The figure shows three views and two pictorial views of one solid part (mm, origin at its lowest corner). Answer the questions. A direction names the side the tool comes from. Round coordinates to 2 decimals unless told otherwise and drop trailing zeros. Loops run counter-clockwise (first coordinate to the right, second up) from the corner with the lowest first, then second, coordinate; pieces in that order, holes last. Notation, with made-up numbers: (-27.5, -33.75) -> (13.5, -33.75) arc R33 ccw to (13.5, -4.75) -> close; hole circle Ø1 at (36, 14). An arc over 180 degrees is marked (long way). Put each result on its own line as item: value.
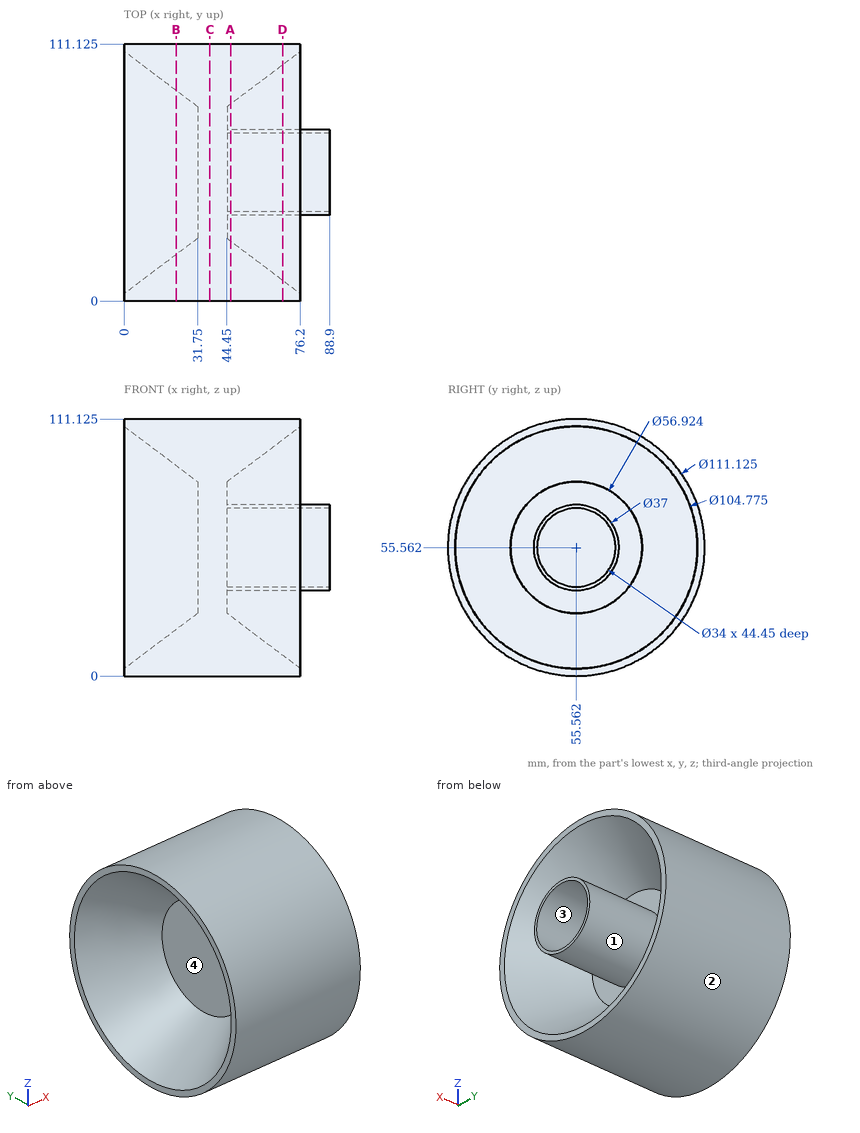
Item 1: The part is cut by section B-B (x = 22.5). Determine the outline of the cut face in (y, z) (1 decimal).
Derived:
outline: circle Ø111.1 at (55.6, 55.6); hole circle Ø70.9 at (55.6, 55.6)
Item 2: The part is cut by section A-A (x = 46). Determine the outline of the cut face in (y, z) (1 decimal), then the cut area to 3 significant figures.
Derived:
outline: circle Ø111.1 at (55.6, 55.6); circle Ø37 at (55.6, 55.6); hole circle Ø59.3 at (55.6, 55.6); hole circle Ø34 at (55.6, 55.6)
area: 7,110 mm^2
Item 3: For a pull along Z with two mould halves and no side action, classify the marked faces 1 and 2 as pulls with the +Z half, pulls with the -Z half, needs draft (parallel to the pull), parting line crosses it, or undercut.
Derived:
face 1: undercut
face 2: parting line crosses it
Item 4: The part is cut by section D-D (x = 68.5). Determine the outline of the cut face in (y, z) (1 decimal), then the cut area to 3 significant figures.
Derived:
outline: circle Ø111.1 at (55.6, 55.6); circle Ø37 at (55.6, 55.6); hole circle Ø93.2 at (55.6, 55.6); hole circle Ø34 at (55.6, 55.6)
area: 3,050 mm^2
Item 5: Which of the six approach directions +Z, -Z, +X, -X, +Y, -Y give full straight-line access (tool end or side, diameter ignored) to the marked faces 3 and 4?
Derived:
face 3: +X
face 4: -X
Item 6: Flat-ended cylindrical pins translate along their axes: pin 1 Ø12 at (x, y) = (14.5, 18) entering from +Z; pin 2 Ø8 at (y, z) = (55.5, 94) entering from +X (1 decimal); pin 3 Ø5 at (y, z) = (58, 73.5) entering from -X. Find the tip coordinate at first contact, or state that the pin passes through.
Derived:
pin 1: stops at z = 101.29
pin 2: stops at x = 63
pin 3: stops at x = 31.75
Item 7: The part is cut by section C-C (x = 37). Determine the outline of the cut face in (y, z) (1 decimal).
Derived:
outline: circle Ø111.1 at (55.6, 55.6)
Item 8: Find the intervals of material crossed by line 1 along Z through (x, y) = (75, 41.5) (1 decimal); line 2 along X through (y, z) = (82, 48.5); line 3 along Y through (x, z) = (83, 60), in increasing order.
Derived:
line 1: z = 1.8 to 6, 43.5 to 46, 65.1 to 67.6, 105.1 to 109.3
line 2: x = 31.75 to 44.45
line 3: y = 37.6 to 39.15, 71.97 to 73.52
